from build123d import *

# Parameters (mm, degrees)
F0_W         = 18.5
F0_H         = 11
F1_DEPTH     = 9.25
F2_DEPTH     = 9.25
F3_R         = 19
F5_DEPTH     = 25.4
F6_DEPTH     = 25.4
F4_R         = 19
F7_DEPTH     = 25.4
F8_DEPTH     = 25.4
F9_R         = 4
F10_DEPTH    = 3.45753
F11_DEPTH    = 7.5
F12_T1_DEPTH = 36
F13_R        = 0.7
F14_R        = 0.5


# Not quite as in the source:
# - a fillet or chamfer that OpenCascade refuses, or shapes differently, is made with other operations: its cross-section is extruded or revolved along the edge and cut away or added
# - a feature names something its author has since deleted; it is built from what else it names


with BuildPart() as f1:
    # F0 (on Front) → F1 (new body)
    with BuildSketch(Plane.XZ):
        Rectangle(F0_W, F0_H)
    extrude(amount=-F1_DEPTH)

    # F0 (on Front) → F2 (join)
    with BuildSketch(Plane.XZ):
        Rectangle(F0_W, F0_H)
    extrude(amount=F2_DEPTH)

    # F3 (on Front) → F5 (cut)
    with BuildSketch(Plane.XZ):
        with Locations((0, -22.5)):
            Circle(F3_R)
    extrude(amount=-F5_DEPTH, mode=Mode.SUBTRACT)

    # F3 (on Front) → F6 (cut)
    with BuildSketch(Plane.XZ):
        with Locations((0, -22.5)):
            Circle(F3_R)
    extrude(amount=F6_DEPTH, mode=Mode.SUBTRACT)

    # F4 (on Right) → F7 (cut)
    with BuildSketch(Plane.YZ):
        with Locations((0, -22.5)):
            Circle(F4_R)
    extrude(amount=-F7_DEPTH, mode=Mode.SUBTRACT)

    # F4 (on Right) → F8 (cut)
    with BuildSketch(Plane.YZ):
        with Locations((0, -22.5)):
            Circle(F4_R)
    extrude(amount=F8_DEPTH, mode=Mode.SUBTRACT)

    # F9 (on face) → F10 (join)
    with BuildSketch(Plane(origin=(0, 0, -5.5), x_dir=(1, 0, 0), z_dir=(0, 0, -1))):
        Circle(F9_R)
    extrude(amount=-F10_DEPTH)

    # F11 (add): a face of the model
    f11_faces = [f1.faces().sort_by_distance(p)[0] for p in [
        (0, 0, -5.5),
    ]]
    extrude(f11_faces, amount=F11_DEPTH)

    # F12: fillet of radius 5 on 4 edges, made by hand

    # F12_s2 → F12_t1 (cut)
    with BuildSketch(Plane.XY.offset(-18)):
        with BuildLine():
            ThreePointArc((-9.25, -4.25), (-7.7855339059, -7.7855339059), (-4.25, -9.25))
            Line((-4.25, -9.25), (-9.25, -9.25))
            Line((-9.25, -9.25), (-9.25, -4.25))
        make_face()
        with BuildLine():
            ThreePointArc((-4.25, 9.25), (-7.7855339059, 7.7855339059), (-9.25, 4.25))
            Line((-9.25, 4.25), (-9.25, 9.25))
            Line((-9.25, 9.25), (-4.25, 9.25))
        make_face()
        with BuildLine():
            ThreePointArc((9.25, 4.25), (7.7855339059, 7.7855339059), (4.25, 9.25))
            Line((4.25, 9.25), (9.25, 9.25))
            Line((9.25, 9.25), (9.25, 4.25))
        make_face()
        with BuildLine():
            ThreePointArc((9.25, -4.25), (7.7855339059, -7.7855339059), (4.25, -9.25))
            Line((4.25, -9.25), (9.25, -9.25))
            Line((9.25, -9.25), (9.25, -4.25))
        make_face()
    extrude(amount=F12_T1_DEPTH, mode=Mode.SUBTRACT)

    # F13
    f13_edges = [f1.edges().sort_by_distance(p)[0] for p in [
        (9.25, 0, 5.5),
        (7.785534, -7.785534, 5.5),
        (0, -9.25, 5.5),
        (-7.785534, -7.785534, 5.5),
        (-9.25, 0, 5.5),
        (-7.785534, 7.785534, 5.5),
        (0, 9.25, 5.5),
        (7.785534, 7.785534, 5.5),
    ]]
    fillet(f13_edges, radius=F13_R)

    # F14
    f14_edges = [f1.edges().sort_by_distance(p)[0] for p in [
        (-4, 0, -13),
    ]]
    fillet(f14_edges, radius=F14_R)


solid = f1.part
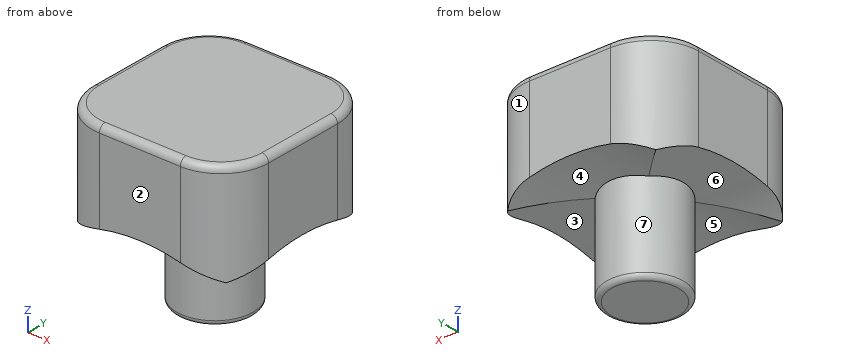
Part model, mm, in its own coordinate system. Face numbers are marked on the shaded views. A direction names the side the tool comes from. Coordinates: 2 decimals unless noted, no trailing zeros. Loops run counter-clockwise (first coordinate to the right, second up) from the corner with the lowest first, then second, coordinate; pieces in that order, holes last. Notation, with made-up numbers: (34, 54) -> (71, 54) arc R18 cw to (71, 62) -> close; hole circle Ø11 at (89.25, -5.5). An arc over 180 degrees is marked (long way). Use a Markdown table: item, result. Add a question column.
Item 1: Pull direction Y, two halves, no side cores. Call the marked faces 1, 2 and 3: +Y half, -Y half, draft (parallel to the pull), parting line (faces both ways), or undercut.
Item 2: Flat gauge pins, fed straight in: P1, Ø2, axis at x = -1.5, z = -10, coming from the -Y side; P2, Ø1.5, axis at x = 7, z = -3, coming from the +Y side. Where does each tip first touch, or does it go through?
Item 3: Which spindle directions (+Z, -Z, +X, -X, +Y, -Y) get a long thin tool onto all of the face, cutting with end or side? Do the marked faces 4, 5, 6 and 7. Say none if no direction does.
Item 4: Probe probe 1 along Z at (x, y) = (-7.5, 0.25); probe 2 along Z at (x, y) = (4.25, 4.25); probe 3 along X at (y, z) = (-2.5, -7.75). List the from-to ranges inside material, lowest first.
Item 5: Band-saw the part on D-D on z = -9.5. Write the cut outline in (x, y), plus the area to 3 significant figures.
Item 6: Band-saw the part on A-A on y = 0. Write the cut outline in (x, z).
Item 7: Band-saw the part on C-C on z = 4.25. Write the cut outline in (x, y).
Geometry says:
| question | item | result |
|---|---|---|
| 1 | face 1 | +Y half |
| 1 | face 2 | -Y half |
| 1 | face 3 | undercut |
| 2 | P1 | y = -3.97 |
| 2 | P2 | y = 8.83 |
| 3 | face 4 | -Z, +Y |
| 3 | face 5 | -Z, -Y |
| 3 | face 6 | -Z, -X |
| 3 | face 7 | -Z |
| 4 | probe 1 | -3.5 to 5.5 |
| 4 | probe 2 | -3.98 to 5.5 |
| 4 | probe 3 | -3.12 to 3.12 |
| 5 | outline | circle Ø8 at (0, 0) |
| 5 | area | 50.3 mm² |
| 6 | outline | (-9.25, -3.5) -> (-4, -3.5) -> (-4, -12.5) arc R0.5 ccw to (-3.5, -13) -> (3.5, -13) arc R0.5 ccw to (4, -12.5) -> (4, -3.5) -> (9.25, -3.5) -> (9.25, 4.8) arc R0.7 ccw to (8.55, 5.5) -> (-8.55, 5.5) arc R0.7 ccw to (-9.25, 4.8) -> close |
| 7 | outline | (-9.25, -4.25) arc R5 ccw to (-4.25, -9.25) -> (4.25, -9.25) arc R5 ccw to (9.25, -4.25) -> (9.25, 4.25) arc R5 ccw to (4.25, 9.25) -> (-4.25, 9.25) arc R5 ccw to (-9.25, 4.25) -> close |
